Build history of the part. All positions in model axes, mm. A direction names the side the tool comes from. Coordinates: 2 decimals unless noted, no trailing zeros. Loops run counter-clockwise (first coordinate to the right, second up) from the corner with the lowest first, then second, coordinate; pieces in that order, holes last.
(1) Tool access for faces 4 (the face through (-57.6, -213.01, -17.07)), 5 (the face through (68, -216, -12)): list every direction of +Z, -Z, +X, -X, +Y, -Y with a clear straight run to the whole face (end or side of a thin tool).
(2) Flat gauge pins, fed straight in: P1, Ø1, axis at y = -65, z = -9, coming from the -X side; P2, Ø3, axis at x = 132, z = -5.5, coming from the +Y side; P3, Ø8, axis at x = -219.5, y = -42.5, coming from the +Z side; P4, Ø6.5, axis at x = 167.21, y = -150.55, coming from the -Z side. Where does each tip first touch, or does it go through?
(3) Two-plate mould, pull along X, no slides. Class faces 1 (the face through (74.76, -218.87, -6.08)), 2 (the face through (250, -30, -6)), 3 (the face through (-270, -15, -11)): pulls with the +X half, pulls with the -X half, needs draft (parallel to the pull), parting line crosses it, or undercut.
(4) Wall check: L1, parallel to X at y = -220, z = -20; L2, parallel to X at y = -50.5, z = -9.75; L3, parallel to X at y = -148, z = -15.5. Give the ranges that are in metal, low to high.
(5) Slice it at B-B (x = 0). Give the cut face in (y, z), and give its area (3 significant figures).
(6) Slice it at A-A (y = -60.5). Give the cut face in (x, z).
Autodesk Inventor part; units mm, degrees
ref_plane "YZ Plane" through (0, 0, 0) normal (1, 0, 0) x (0, 1, 0)
ref_plane "XZ Plane" through (0, 0, 0) normal (0, 1, 0) x (-1, 0, 0)
ref_plane "XY Plane" through (0, 0, 0) normal (0, 0, 1) x (1, 0, 0)
sketch "Sketch1" plane through (0, 0, 0) normal (0, 0, 1) x (1, 0, 0)
  circle A0 centre (0, 0) radius 220 construction
  circle A1 centre (0, 0) radius 205
  circle A2 centre (0, 0) radius 240
  line L0 (-205, 0) -> (-205, 80) construction
  line L1 (-205, 80) -> (-240, 80) construction
  line L2 (-240, 80) -> (-240, 0) construction
  line L3 (-205, 0) -> (-240, 0)
  line L4 (-240, 0) -> (-270, 0)
  line L5 (-270, 0) -> (-270, -30)
  line L6 (-270, -30) -> (-238.1176, -30)
  line L7 (-1.5, -238) -> (1.5, -238)
  line L8 (1.5, -238) -> (1.5, -280)
  line L9 (1.5, -280) -> (-1.5, -280)
  line L10 (-1.5, -280) -> (-1.5, -238)
  line L11 (0, -238) -> (0, -205)
  line L12 (-1.5, -280) -> (-30, -280)
  line L13 (-30, -280) -> (-30, -238.1176)
  line L14 (0, -238) -> (0, -240)
  point P0 (0, -280)
  point P1 (-1.5, -239.9953)
  point P2 (1.5, -239.9953)
  dimension "d26" = 80
  dimension "d40" = 30
  dimension "d41" = 30
  dimension "d74" = 410
  dimension "d75" = 3
  dimension "d76" = 42
  dimension "d77" = 30
  dimension "d78" = 2
  dimension "d98" = 480
  dimension "d99" = 440
extrude "Extrusion1" add sketch "Sketch1" against normal blind 22 contours A1 L11 L7 L10 A2 L3 | A2 L6 L5 L4 | L14 A2 L10 L7
sketch "Sketch10" plane through (-270, -30, 0) normal (0, -1, 0) x (1, 0, 0)
  line L0 (0, 0) -> (31.8824, 0)
  line L1 (0, 0) -> (0, -22)
  line L2 (31.8824, -22) -> (0, -22)
  line L3 (31.8824, 0) -> (31.8824, -22)
  circle A0 centre (15.9412, -11) radius 5.5
  line L4 (0, 0) -> (0, -22)
  line L5 (0, 0) -> (31.8824, 0)
  point P0 (270, 0)
  point P1 (0, -11)
  point P2 (15.9412, 0)
  dimension "d79" = 11
extrude "Extrusion9" cut sketch "Sketch10" against normal through all contours A0
mirror "Mirror3" about plane through (0, 0, 0) normal (1, 0, 0) of "Extrusion1", "Extrusion9"
sketch "Sketch12" plane through (0, 0, 0) normal (0, 0, 1) x (1, 0, 0)
  line L0 (0, 0) -> (-225, 0) construction
  line L1 (0, 0) -> (-221.5817, -39.0708) construction
  circle A0 centre (0, 0) radius 225 construction
  dimension "d86" = 10
  dimension "d87" = 450
hole "Hole4" at (-221.5817, -39.0708, 0) direction (0, 0, -1) diameter 11 end through all counterbore diameter 26 counterbore depth 12
pattern_circular "Circular Pattern5" count 6 over 160 about axis through (0, 0, -10) along (0, 0, 1) of "Hole4"
equation "\"d41\" = d40"
equation "\"d93\" = Thickness"
equation "\"BendReliefDepth\" = 0.5 * Thickness"
properties part number "ДМФ 093 Постель КОРМА v2.0_CPY" material "Nylon 6"
Response values:
1. face 4: +Z, -Z
1. face 5: +Z
2. P1: stops at x = -231.17
2. P2: stops at y = -155.57
2. P3: stops at z = -12
2. P4: passes through
3. face 1: undercut
3. face 2: needs draft
3. face 3: pulls with the -X half
4. L1: x = -95.92 to -66.07, -57.96 to 57.96, 66.07 to 95.92
4. L2: x = -234.63 to -227.78, -215.39 to -198.68, 198.68 to 215.39, 227.78 to 234.63
4. L3: x = -188.93 to -172.08, -162.34 to -141.85, 141.85 to 162.34, 172.08 to 188.93
5. outline: (-240, -22) - (-205, -22) - (-205, 0) - (-240, 0) - close
5. area: 770 mm2
6. outline: (-232.25, -22) - (-195.87, -22) - (-195.87, 0) - (-232.25, 0) - close; (195.87, -22) - (232.25, -22) - (232.25, 0) - (195.87, 0) - close
